Read the model definition and answer for the solid it produces. Units are mm, in the model's axes. A direction names the side the tool comes from. Give positions to 0.01 mm unless a question says otherwise; leave off trailing zeros. Loops run counter-clockwise (first coordinate to the right, second up) from the corner with the lowest first, then second, coordinate; pieces in that order, holes last. Notation, with made-up numbers: (4.25, 12.25) -> (11.25, 12.25) arc R23 cw to (11.25, 37.25) -> close; hole circle Ø7 at (9.25, 70.5). An arc over 180 degrees is marked (long way). One line per item, written item: value. Start each with the question number.
from build123d import *

# Parameters (mm, degrees)
F0_W     = 20.157362
F0_H     = 20.157362
F1_DEPTH = 1.1
F2_R     = 2.529732
F2_R_2   = 2.415473
F2_R_3   = 2.705087
F3_DEPTH = 1.6


with BuildPart() as f1:
    # F0 (on Top) → F1 (new body)
    with BuildSketch(Plane.XY):
        with Locations((-3.302667, 0.387924)):
            Rectangle(F0_W, F0_H)
    extrude(amount=F1_DEPTH)

    # F2 (on face) → F3 (join)
    with BuildSketch(Plane.XY.offset(1.1)):
        with Locations((-8.835531, 5.941908)):
            Circle(F2_R)
        with Locations((1.701719, 6.566437)):
            Circle(F2_R_2)
        with Locations((-9.036944, -4.364801)):
            Circle(F2_R_3)
    extrude(amount=F3_DEPTH)


solid = f1.part
Item 1: Section D-D, the plane y = -2 is taken. Determine the outline of the cut face in (x, z).
Item 2: Section B-B, the plane z = 2.2 is taken. Determine the outline of the cut face in (x, y), plus the area to 3 significant figures.
Item 3: Section A-A, the plane y = 5.5 is taken. Determine the outline of the cut face in (x, z).
Item 4: Consider L1, parallel to Z at x = 1.5, y = -3.25; L2, parallel to Y at x = 2.5, z = 2.55; L3, parallel to X at y = -3, z = 2.25. Determine where each line is inside the solid, lowest interval first. Write a range as [from, to].
Item 5: Section C-C, the plane x = 3 is taken. Determine the outline of the cut face in (y, z), plus the area to 3 significant figures.
Item 6: For faces 1 (the flat face through (2, 7, 2.7)), 2 (the cylindrical face through (-6.457, -3.552, 1.889)), determine the directions among +Z, -Z, +X, -X, +Y, -Y from which every point of the face is accessible in a straight line to the end or side of a thin tool.
Item 7: Determine the mould class of faces 3 (the cylindrical face through (1.39, 8.96, 1.89)), 4 (the flat face through (-13.381, 0.2, 0.5)), 5 (the flat face through (-3.4, -9.691, 0.5)), 6 (the flat face through (6.776, 0.2, 0.5)) for opening direction X: pulls with the +X half, pulls with the -X half, needs draft (parallel to the pull), parting line crosses it, or undercut.
Computed values:
1. outline: (-13.38, 0) -> (6.78, 0) -> (6.78, 1.1) -> (-7.72, 1.1) -> (-7.72, 2.7) -> (-10.35, 2.7) -> (-10.35, 1.1) -> (-13.38, 1.1) -> close
2. outline: circle Ø5.41 at (-9.04, -4.36); circle Ø5.06 at (-8.84, 5.94); circle Ø4.83 at (1.7, 6.57)
2. area: 61.4 mm²
3. outline: (-13.38, 0) -> (6.78, 0) -> (6.78, 1.1) -> (3.87, 1.1) -> (3.87, 2.7) -> (-0.47, 2.7) -> (-0.47, 1.1) -> (-6.34, 1.1) -> (-6.34, 2.7) -> (-11.33, 2.7) -> (-11.33, 1.1) -> (-13.38, 1.1) -> close
4. L1: [0, 1.1]
4. L2: [4.29, 8.85]
4. L3: [-11.37, -6.7]
5. outline: (-9.69, 0) -> (10.47, 0) -> (10.47, 1.1) -> (8.6, 1.1) -> (8.6, 2.7) -> (4.53, 2.7) -> (4.53, 1.1) -> (-9.69, 1.1) -> close
5. area: 28.7 mm²
6. face 1: +Z, +X, -X, +Y, -Y
6. face 2: +Z
7. face 3: undercut
7. face 4: pulls with the -X half
7. face 5: needs draft
7. face 6: pulls with the +X half
